from build123d import *

# Parameters (mm, degrees)
F1_DEPTH = 6
F2_D     = 3.3
F3_D     = 6


with BuildPart() as f1:
    # F0 (on Top) → F1 (new body)
    with BuildSketch(Plane.XY):
        with BuildLine():
            ThreePointArc((25, 28.5), (23.5355339059, 32.0355339059), (20, 33.5))
            Line((20, 33.5), (-20, 33.5))
            ThreePointArc((-20, 33.5), (-23.5355339059, 32.0355339059), (-25, 28.5))
            Line((-25, 28.5), (-25, -28.5))
            ThreePointArc((-25, -28.5), (-23.5355339059, -32.0355339059), (-20, -33.5))
            Line((-20, -33.5), (20, -33.5))
            ThreePointArc((20, -33.5), (23.5355339059, -32.0355339059), (25, -28.5))
            Line((25, -28.5), (25, 28.5))
        make_face()
    extrude(amount=F1_DEPTH)

    # F2 (through all)
    with Locations(Plane(origin=(0, 0, 0), x_dir=(1, 0, 0), z_dir=(0, 0, -1))):
        with Locations((-15, 0), (15, 0)):
            Hole(F2_D / 2)

    # F3 (through all)
    with Locations(Plane(origin=(0, 0, 0), x_dir=(1, 0, 0), z_dir=(0, 0, -1))):
        with Locations((-15, -23.5), (15, 23.5)):
            Hole(F3_D / 2)


solid = f1.part
Could you check a few things on this model? Use its own coordinates, in mm. Coordinates: 2 decimals unless noted, no trailing zeros. Write each loop counter-clockwise with the first axis right and the second up, starting at its lowest first coordinate (ties: lowest second). Pieces come first, ordered by that corner, then holes. Notation, with made-up numbers: (37, 77) - (44, 77) arc R21 cw to (44, 98) - close; hole circle Ø10 at (41.25, -21.5). An arc over 180 degrees is marked (long way). Write item = value, one per line.
1) We'd pull the mould along Y, two halves only. Please class faces 1 (the flat face through (-25, 0, 3)), 2 (the cylindrical face through (23.5, -32.07, 2.96)), 3 (the cylindrical face through (13.476, 0.632, 3.042)), 4 (the cylindrical face through (-12.6, 25.3, 3)): +Y half, -Y half, draft (parallel to the pull), parting line (faces both ways), or undercut.
Result set:
face_1 = draft
face_2 = -Y half
face_3 = undercut
face_4 = undercut
2) Suppose I cut it at C-C on y = 0. Please give me the cut outline in (x, z), plus the area to 3 significant figures.
Result set:
outline = (-25, 0) - (-16.65, 0) - (-16.65, 6) - (-25, 6) - close; (-13.35, 0) - (13.35, 0) - (13.35, 6) - (-13.35, 6) - close; (16.65, 0) - (25, 0) - (25, 6) - (16.65, 6) - close
area = 260 mm2
3) Will this pin go through, and if not, where does the flat tip stop? pin 1 Ø9.5 at (x, y) = (-15, 23.5) entering from -Z.
Result set:
pin_1 = 0
4) Suppose I cut it at B-B on x = -15. Please give me the cut outline in (y, z).
Result set:
outline = (-33.5, 0) - (-1.65, 0) - (-1.65, 6) - (-33.5, 6) - close; (1.65, 0) - (20.5, 0) - (20.5, 6) - (1.65, 6) - close; (26.5, 0) - (33.5, 0) - (33.5, 6) - (26.5, 6) - close
5) Suppose I cut it at A-A on y = -23.5. Please give me the cut outline in (x, z).
Result set:
outline = (-25, 0) - (12, 0) - (12, 6) - (-25, 6) - close; (18, 0) - (25, 0) - (25, 6) - (18, 6) - close
6) Suppose I cut it at D-D on z = 4.75. Please give me the cut outline in (x, y), plus the area to 3 significant figures.
Result set:
outline = (-25, -28.5) arc R5 ccw to (-20, -33.5) - (20, -33.5) arc R5 ccw to (25, -28.5) - (25, 28.5) arc R5 ccw to (20, 33.5) - (-20, 33.5) arc R5 ccw to (-25, 28.5) - close; hole circle Ø6 at (-15, 23.5); hole circle Ø3.3 at (-15, 0); hole circle Ø6 at (15, -23.5); hole circle Ø3.3 at (15, 0)
area = 3,250 mm2
7) Please list where these lines run through material, in increasing order: line 1 (Y direction, x = -15, z = 1.45); line 2 (X direction, y = 23.5, z = 3.8); line 3 (Y direction, x = 15, z = 1.8). Write a range as [from, to].
Result set:
line_1 = [-33.5, -1.65], [1.65, 20.5], [26.5, 33.5]
line_2 = [-25, -18], [-12, 25]
line_3 = [-33.5, -26.5], [-20.5, -1.65], [1.65, 33.5]
